```python
from build123d import *

# Parameters (mm, degrees)
CROQUIS1_R              = 17.5
SALIENTE_EXTRUIR1_DEPTH = 7.5
CROQUIS2_R              = 17.5
CROQUIS2_R_2            = 15
CORTAR_EXTRUIR1_DEPTH   = 5
CROQUIS3_R              = 1.5
CORTAR_EXTRUIR2_DEPTH   = 10


with BuildPart() as part:
    # Croquis1 → Saliente-Extruir1 (new, symmetric)
    with BuildSketch(Plane(origin=(0, 0, 0), x_dir=(0, 1, 0), z_dir=(0, 0, 1))):
        with Locations(Location((0, 0, 0), (0, 0, 270))):
            Circle(CROQUIS1_R)
    extrude(amount=SALIENTE_EXTRUIR1_DEPTH, both=True)

    # Croquis2 → Cortar-Extruir1 (cut, symmetric)
    with BuildSketch(Plane(origin=(0, 0, 0), x_dir=(0, 1, 0), z_dir=(0, 0, 1))):
        with Locations(Location((0, 0, 0), (0, 0, 270))):
            Circle(CROQUIS2_R)
        with Locations(Location((0, 0, 0), (0, 0, 270))):
            Circle(CROQUIS2_R_2, mode=Mode.SUBTRACT)
    extrude(amount=CORTAR_EXTRUIR1_DEPTH, both=True, mode=Mode.SUBTRACT)

    # Croquis3 → Cortar-Extruir2 (cut, symmetric)
    with BuildSketch(Plane(origin=(0, 0, 0), x_dir=(0, 1, 0), z_dir=(0, 0, 1))):
        with Locations(Location((6, 0, 0), (0, 0, 270))):
            Circle(CROQUIS3_R)
        with Locations(Location((-6, 0, 0), (0, 0, 270))):
            Circle(CROQUIS3_R)
    extrude(amount=CORTAR_EXTRUIR2_DEPTH, both=True, mode=Mode.SUBTRACT)


solid = part.part
```
Input: part model. Units: mm. Frame: model coordinates. A direction names the side the tool comes from. Coordinates: 2 decimals unless noted, no trailing zeros. Order: outer loops, then holes, each group sorted by start corner. A loop starts at its lowest first (then second) coordinate and runs counter-clockwise, first axis right, second up. Notation, with made-up numbers: (53.5, 20.5) - (83.5, 20.5) arc R19 ccw to (83.5, 52.5) - close; hole circle Ø11 at (40, 85.5). An arc over 180 degrees is marked (long way). Put each result on its own line as item: value.
1. Contact query for flat-ended pins moving along their axis: pin 1 Ø2.5 at (x, y) = (0, 6) entering from -Z; pin 2 Ø1.5 at (y, z) = (-10.5, 1) entering from -X; pin 3 Ø4 at (x, z) = (10, 2.5) entering from +Y; pin 4 Ø3 at (y, z) = (12, 0.5) entering from -X. Output: stop coordinate, or through.
Report:
pin 1: passes through
pin 2: stops at x = -11.4
pin 3: stops at y = 12.69
pin 4: stops at x = -10.71
2. Cut plane D-D on y = 0. Return the cut outline in (x, z), then the cut area to 3 significant figures.
Report:
outline: (-17.5, -7.5) - (17.5, -7.5) - (17.5, -5) - (15, -5) - (15, 5) - (17.5, 5) - (17.5, 7.5) - (-17.5, 7.5) - (-17.5, 5) - (-15, 5) - (-15, -5) - (-17.5, -5) - close
area: 475 mm2
3. Cut plane A-A on x = 0. Return the cut outline in (y, z).
Report:
outline: (-17.5, -7.5) - (-7.5, -7.5) - (-7.5, 7.5) - (-17.5, 7.5) - (-17.5, 5) - (-15, 5) - (-15, -5) - (-17.5, -5) - close; (-4.5, -7.5) - (4.5, -7.5) - (4.5, 7.5) - (-4.5, 7.5) - close; (7.5, -7.5) - (17.5, -7.5) - (17.5, -5) - (15, -5) - (15, 5) - (17.5, 5) - (17.5, 7.5) - (7.5, 7.5) - close
4. Cut plane C-C on z = -1.5. Return the cut outline in (x, y), then the cut area to 3 significant figures.
Report:
outline: circle Ø30 at (0, 0); hole circle Ø3 at (0, -6); hole circle Ø3 at (0, 6)
area: 693 mm2
5. Cut plane B-B on y = -7. Return the cut outline in (x, z), then the cut area to 3 significant figures.
Report:
outline: (-16.04, -7.5) - (-1.12, -7.5) - (-1.12, 7.5) - (-16.04, 7.5) - (-16.04, 5) - (-13.27, 5) - (-13.27, -5) - (-16.04, -5) - close; (1.12, -7.5) - (16.04, -7.5) - (16.04, -5) - (13.27, -5) - (13.27, 5) - (16.04, 5) - (16.04, 7.5) - (1.12, 7.5) - close
area: 392 mm2
6. Reachability of faces 1 (the face through (13, 8, -5)), 2 (the face through (-13.887, -10.648, -6.232)) from +Z, -Z, +X, -X, +Y, -Y: full face, straight path, thin tool, end or side. Return the list, or none.
Report:
face 1: none
face 2: +Z, -Z
7. Draft query along Y for faces 3 (the face through (-13.887, -10.648, 6.268)), 4 (the face through (0.69, -7.33, 0.11)), 5 (the face through (0, 0, -7.5)), 6 (the face through (0.69, 4.67, 0.11)). Return one class per face: pulls with the +Y half, pulls with the -Y half, needs draft (parallel to the pull), parting line crosses it, or undercut.
Report:
face 3: parting line crosses it
face 4: undercut
face 5: needs draft
face 6: undercut
8. Line query: line 1 along Y through (x, z) = (0, -4); line 2 along X through (y, z) = (0.5, -3); line 3 along Y through (x, z) = (1, 1.5). Output: solid intervals per line, ascending.
Report:
line 1: y = -15 to -7.5, -4.5 to 4.5, 7.5 to 15
line 2: x = -14.99 to 14.99
line 3: y = -14.97 to -7.12, -4.88 to 4.88, 7.12 to 14.97
